Check sheet for the modelled part. Datum: model origin and axes. Units: mm. Give positions to 0.01 mm unless a question says otherwise; leave off trailing zeros. Order: outer loops, then holes, each group sorted by start corner. A loop starts at its lowest first (then second) coordinate and runs counter-clockwise, first axis right, second up.
Autodesk Inventor part; units mm, degrees
ref_plane "YZ Plane" through (0, 0, 0) normal (1, 0, 0) x (0, 1, 0)
ref_plane "XZ Plane" through (0, 0, 0) normal (0, 1, 0) x (-1, 0, 0)
ref_plane "XY Plane" through (0, 0, 0) normal (0, 0, 1) x (1, 0, 0)
sketch "Sketch1" plane through (0, 0, 0) normal (0, 1, 0) x (-1, 0, 0)
  line L0 (0, 0) -> (-710, 0)
  line L1 (-710, 0) -> (-710, -150)
  line L2 (-710, -150) -> (0, -150)
  line L3 (0, -150) -> (0, 0)
  dimension "d0" = 710
  dimension "d1" = 150
extrude "Extrusion1" add sketch "Sketch1" along normal blind 1.6
sketch "Sketch2" plane through (0, 1.6, 0) normal (0, 1, 0) x (1, 0, 0)
  line L0 (710, 0) -> (690, 0)
  line L1 (690, 0) -> (690, 60)
  line L2 (690, 60) -> (710, 60)
  line L3 (710, 60) -> (710, 0)
  circle A0 centre (700, 80) radius 2.5
  circle A1 centre (700, 130) radius 2.5
  line L4 (710, 150) -> (0, 150)
  point P0 (0, 0)
  point P1 (700, 60)
  dimension "d6" = 20
  dimension "d7" = 60
  dimension "d10" = 5
  dimension "d11" = 5
  dimension "d12" = 50
  dimension "d13" = 20
extrude "Extrusion3" cut sketch "Sketch2" against normal blind 1.6
sketch "Sketch3" plane through (690, 1.6, 0) normal (1, 0, 0) x (0, 0, -1)
  line L0 (0, -1.6) -> (54, -1.6)
  line L1 (54, -1.6) -> (54, 0)
  line L2 (54, 0) -> (0, 0)
  line L3 (0, 0) -> (0, -1.6)
  dimension "d16" = 54
  dimension "d17" = 1.6
extrude "Extrusion4" add sketch "Sketch3" along normal blind 95
properties part number "X-Axis Panel Left" material "Steel"
(1) Cross-section at A-A on y = 1.2. Enter the section's corners in (x, z), then the cut area to 3 significant figures.
Response values:
outline: (0, -150) - (710, -150) - (710, -60) - (690, -60) - (690, -54) - (785, -54) - (785, 0) - (0, 0) - close; hole circle Ø5 at (700, -130); hole circle Ø5 at (700, -80)
area: 110,000 mm2
(2) Gauge pin test, flat ends, axial feed: pin 1 Ø4.5 at (x, z) = (700, -130) entering from -Y; pin 2 Ø0.8 at (x, y) = (756.5, 0.5) entering from -Z. Record the tip position at first contact, or that the pin passes through.
Response values:
pin 1: passes through
pin 2: stops at z = -54
(3) Material ranges on L1, parallel to Z at x = 700, y = 0.6; L2, parallel to X at y = 1.25, z = -130; L3, parallel to Z at x = 699, y = 1.3, recorded low to high.
Response values:
L1: z = -150 to -132.5, -127.5 to -82.5, -77.5 to -60, -54 to 0
L2: x = 0 to 697.5, 702.5 to 710
L3: z = -150 to -132.29, -127.71 to -82.29, -77.71 to -60, -54 to 0
